```python
from build123d import *

# Parameters (mm, degrees)
F3_DEPTH = 2.54


with BuildPart() as f1:
    # F0 (on Front) → F1 (revolve)
    with BuildSketch(Plane.XZ):
        Polygon((0, -7.47395), (0, 0), (-2.8702, 0), (-2.8702, -3.5052), (-1.389063, -3.5052), (-1.389063, -7.47395), align=None)
    revolve(axis=Axis((0, 0, -3.736975), (0, 0, -1)))

    # F2 (on face) → F3 (cut)
    with BuildSketch(Plane.XY):
        Polygon((0.801976, 1.389063), (-0.801976, 1.389063), (-1.603951, 0), (-0.801976, -1.389063), (0.801976, -1.389062), (1.603951, 0), align=None)
    extrude(amount=-F3_DEPTH, mode=Mode.SUBTRACT)


solid = f1.part
```
The model under review builds one solid part; all positions refer to its coordinate system, in mm. A direction names the side the tool comes from. Round coordinates to 2 decimals unless told otherwise and drop trailing zeros. Loops run counter-clockwise (first coordinate to the right, second up) from the corner with the lowest first, then second, coordinate; pieces in that order, holes last.
Item 1: Take a section at C-C (z = -6.25). Write out the cut boundary in (x, y), then the cut area to 3 significant figures.
Determined:
outline: circle Ø2.78 at (0, 0)
area: 6.06 mm2
Item 2: Take a section at D-D (y = -1.7). Write out the cut boundary in (x, z), then the cut area to 3 significant figures.
Determined:
outline: (-2.31, -3.51) - (2.31, -3.51) - (2.31, 0) - (-2.31, 0) - close
area: 16.2 mm2
Item 3: Take a section at B-B (y = 0.7). Write out the cut boundary in (x, z), then the cut area to 3 significant figures.
Determined:
outline: (-2.78, -3.51) - (-1.2, -3.51) - (-1.2, -7.47) - (1.2, -7.47) - (1.2, -3.51) - (2.78, -3.51) - (2.78, 0) - (1.2, 0) - (1.2, -2.54) - (-1.2, -2.54) - (-1.2, 0) - (-2.78, 0) - close
area: 22.9 mm2
Item 4: For line 1 (Z direction, x = -0.45, y = -2.45); line 2 (Z direction, x = -0.8, y = 0.65); line 3 (X direction, y = -1.1, z = -0.5), list the stretches that pass through material, from the lowest coordinate up.
Determined:
line 1: z = -3.51 to 0
line 2: z = -7.47 to -2.54
line 3: x = -2.65 to -0.97, 0.97 to 2.65
Item 5: Clearance check with flat-ended pins moving along their axes: pin 1 Ø0.5 at (x, z) = (0.5, -1.5) entering from +Y; pin 2 Ø2 at (y, z) = (2, -5) entering from -X. State where each tip first meets the part, or that it passes through.
Determined:
pin 1: stops at y = 2.86
pin 2: stops at x = -0.96
Item 6: Mouldability with a two-part tool opening along Y and no side actions: class faces 4 (the face through (1.2, -1.2, 0)), 5 (the face through (0, 1.389, -1)), 6 (the face through (2.278, -1.746, -1.777)) as released by +Y, released by -Y, zero draft, split by the parting line, or undercut.
Determined:
face 4: zero draft
face 5: undercut
face 6: split by the parting line
Item 7: Take a section at A-A (x = 0). Write out the cut boundary in (y, z).
Determined:
outline: (-2.87, -3.51) - (-1.39, -3.51) - (-1.39, -7.47) - (1.39, -7.47) - (1.39, -3.51) - (2.87, -3.51) - (2.87, 0) - (1.39, 0) - (1.39, -2.54) - (-1.39, -2.54) - (-1.39, 0) - (-2.87, 0) - close
Item 8: For faces 1 (the face through (-1.2, -0.7, -1.3)), 2 (the face through (0.301, -1.356, -5.517)), 3 (the face through (0, 0, -7.474)), list the 3-axis set-ups (+Z, -Z, +X, -X, +Y, -Y) from which the entire face can be reached by the end or side of a thin tool; tool diameter is ignored.
Determined:
face 1: +Z
face 2: -Z
face 3: -Z, +X, -X, +Y, -Y
